Here's the drawing with two shaded views (mm, measured from the low corner). I have some questions. A direction names the side the tool comes from. Coordinates: 2 decimals unless noted, no trailing zeros. Loops run counter-clockwise (first coordinate to the right, second up) from the corner with the lowest first, then second, coordinate; pieces in that order, holes last. Notation, with made-up numbers: M 54,14 L 106,14 A24 cw 106,34 Z; hole C 71.5,22.5 d10. An arc over 180 degrees is marked long. Return JSON: item names as keys, results as strings. Group by question number.
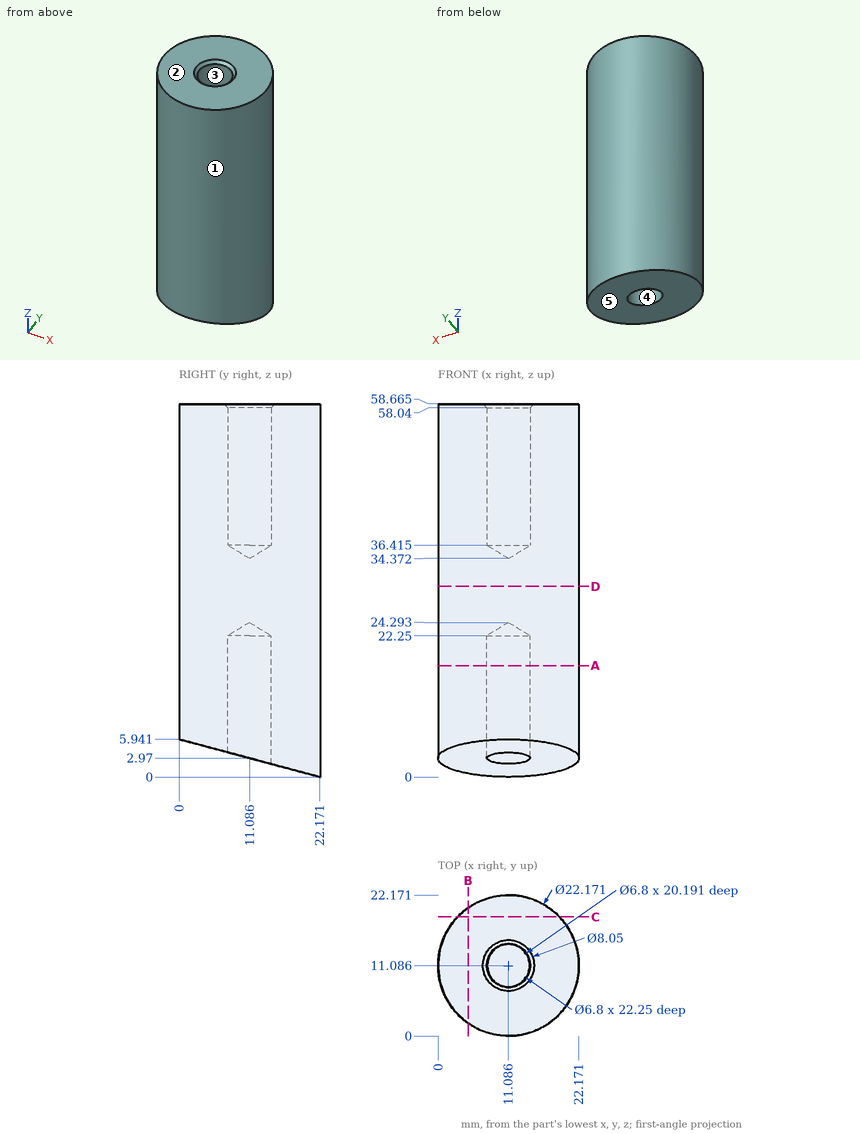
1) Suppose I cut it at C-C, the plane y = 18.75. List the corners of the cut face in (x, z) for me (1 decimal).
2) Suppose I cut it at D-D, the plane z = 30. List the corners of the cut face in (x, y) for me (1 decimal).
3) If I drill on line 1 (Y direction, x = 8.25, z = 39) (1 decimal); line 2 (X direction, y = 10, z = 6.5); line 3 (Y direction, x = 10.5, z = 6.5) (1 decimal), over which ranges is the centre line in solid material (lowest first)? Write a range as from..to.
4) Suppose I cut it at B-B, the plane x = 4.75. List the corners of the cut face in (y, z) for me (1 decimal).
5) For pin 1 (5 mm diameter, centred on x = 14, z = 27.5, fed in from +Y); pin 2 (1.5 mm diameter, centred on y = 9, z = 50, fed in from +X); pin 3 (5.5 mm diameter, centred on x = 11.09, y = 11.09, fed in from -Z); pin 4 (4 mm diameter, centred on y = 12, z = 30, fed in from -X), each with a flat end and sliding along its axis, tell me the tip position at first contact or that it passes through.
6) If we mould it in two halves opening along X, with no side actions, what happens to the marked faces 1, 2 and 3? For each: +X half, -X half, draft (parallel to the pull), parting line (faces both ways), or undercut.
7) Suppose I cut it at A-A, the plane z = 17.5. List the corners of the cut face in (x, y) for me (1 decimal), then the cut area to 3 significant figures.
8) For the marked faces 4 and 5, which set-ups out of +Z, -Z, +X, -X, +Y, -Y let a thin tool reach every point of the face, with its end or its side?
Returned:
{
 "1": {"outline": "M 3.1,0.9 L 19.1,0.9 L 19.1,58.7 L 3.1,58.7 Z"},
 "2": {"outline": "C 11.1,11.1 d22.2"},
 "3": {"line 1": "y = 0.4..9.2, 13..21.8", "line 2": "x = 0.05..7.86, 14.31..22.12", "line 3": "y = 0..7.7, 14.4..22.2"},
 "4": {"outline": "M 2,5.4 L 20.2,0.5 L 20.2,58.7 L 2,58.7 Z"},
 "5": {"pin 1": "stops at y = 22.16", "pin 2": "stops at x = 22.09", "pin 3": "stops at z = 22.64", "pin 4": "stops at x = 0"},
 "6": {"face 1": "parting line", "face 2": "draft", "face 3": "undercut"},
 "7": {"outline": "C 11.1,11.1 d22.2; hole C 11.1,11.1 d6.8", "area": "350 mm²"},
 "8": {"face 4": "-Z", "face 5": "-Z, +X, -X, -Y"}
}
